Model file for the job. Use its own axes, mm. A direction names the side the tool comes from. Give positions to 0.01 mm unless a question says otherwise; leave off trailing zeros. Order: outer loops, then holes, each group sorted by start corner. A loop starts at its lowest first (then second) coordinate and runs counter-clockwise, first axis right, second up. Notation, with made-up numbers: (-20, -1.5) - (31, -1.5) arc R20 ccw to (31, 35.5) - close; hole circle Ø8 at (15, 4.25). An arc over 180 degrees is marked (long way). Return JSON: item names as keys, results as strings. Group by question number.
from build123d import *

# Parameters (mm, degrees)
F0_W     = 52.5
F0_H     = 2.5
F1_DEPTH = 1
F2_W     = 0.5
F2_H     = 2.5
F3_DEPTH = 3
F4_W     = 4
F4_H     = 2
F5_DEPTH = 1


with BuildPart() as f1:
    # F0 (on Right) → F1 (new body)
    with BuildSketch(Plane.YZ):
        Rectangle(F0_W, F0_H)
    extrude(amount=F1_DEPTH)

    # F2 (on face) → F3 (join)
    with BuildSketch(Plane.YZ.offset(1)):
        with Locations((-26, 0)):
            Rectangle(F2_W, F2_H)
        with Locations((26, 0)):
            Rectangle(F2_W, F2_H)
    extrude(amount=F3_DEPTH)

    # F4 (on face) → F5 (cut, through all)
    with BuildSketch(Plane.YZ.offset(1)):
        with Locations((-18.25, 0)):
            Rectangle(F4_W, F4_H)
        with Locations((1.75, 0)):
            Rectangle(F4_W, F4_H)
    extrude(amount=-F5_DEPTH, mode=Mode.SUBTRACT)


solid = f1.part
(1) Slice it at C-C (y = -6). Give the cut face in (x, z), and give its area (3 significant figures).
(2) Slice it at B-B (z = -0.55). Give the cut face in (x, y), and give its area (3 significant figures).
(3) Drop flat-ended pins along their axis: pin 1 Ø1.2 at (y, z) = (-8, 0.5) entering from +X; pin 2 Ø1 at (y, z) = (-5, 0) entering from -X. Give the stop position or say it passes through.
(4) Pull direction Y, two halves, no side cores. Call faces 1 (the face through (0.4, -0.1, 1.25)), 2 (the face through (1, -0.4, 0)), 3 (the face through (2, 26.25, 0)): released by +Y, released by -Y, zero draft, split by the parting line, or undercut.
(5) Drill centre lines: L1, parallel to Y at x = 0.8, z = -0.4; L2, parallel to Z at x = 0.7, y = -19.5; L3, parallel to Y at x = 3.85, z = -0.6. Where is each one in solid material? Low to high.
(6) Slice it at A-A (x = 2.5). Give the cut face in (y, z), and give its area (3 significant figures).
(7) 3-axis set-ups, long thin cutter, end or side, ignore diameter. For faces 4 (the face through (2, 25.75, 0)), 5 (the face through (2, -26.25, 0)), 6 (the face through (0.5, -16.25, 0)): which of +Z, -Z, +X, -X, +Y, -Y reach the whole face in a straight line?
Result set:
{
 "1": {"outline": "(0, -1.25) - (1, -1.25) - (1, 1.25) - (0, 1.25) - close", "area": "2.50 mm²"},
 "2": {"outline": "(0, -26.25) - (4, -26.25) - (4, -25.75) - (1, -25.75) - (1, -20.25) - (0, -20.25) - close; (0, -16.25) - (1, -16.25) - (1, -0.25) - (0, -0.25) - close; (0, 3.75) - (1, 3.75) - (1, 25.75) - (4, 25.75) - (4, 26.25) - (0, 26.25) - close", "area": "47.5 mm²"},
 "3": {"pin 1": "stops at x = 1", "pin 2": "stops at x = 0"},
 "4": {"face 1": "zero draft", "face 2": "undercut", "face 3": "released by +Y"},
 "5": {"L1": "y = -26.25 to -20.25, -16.25 to -0.25, 3.75 to 26.25", "L2": "z = -1.25 to -1, 1 to 1.25", "L3": "y = -26.25 to -25.75, 25.75 to 26.25"},
 "6": {"outline": "(-26.25, -1.25) - (-25.75, -1.25) - (-25.75, 1.25) - (-26.25, 1.25) - close; (25.75, -1.25) - (26.25, -1.25) - (26.25, 1.25) - (25.75, 1.25) - close", "area": "2.50 mm²"},
 "7": {"face 4": "+Z, -Z, +X", "face 5": "+Z, -Z, +X, -X, -Y", "face 6": "+X, -X"}
}
